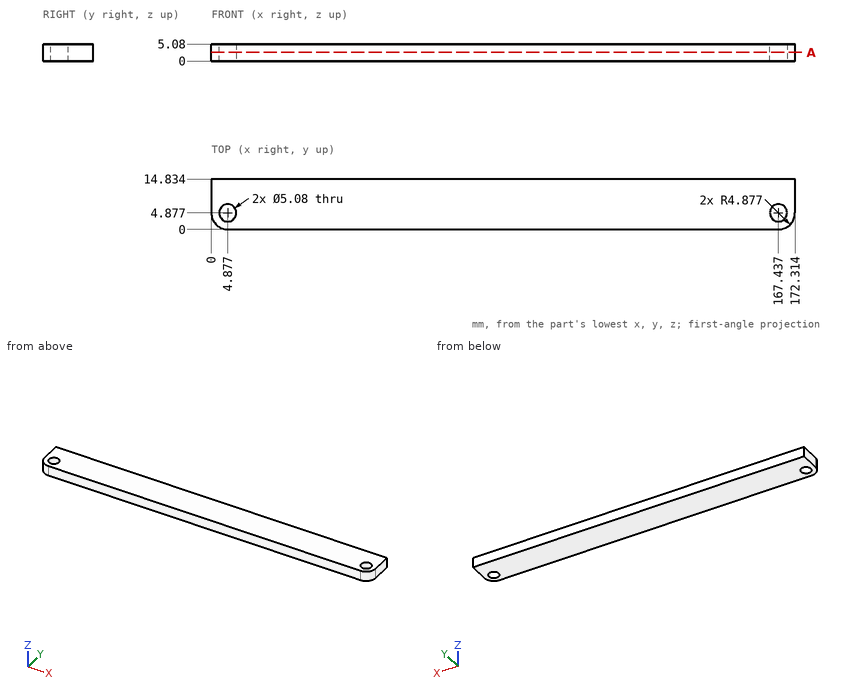
The drawing under review shows one solid part. Ordinate dimensions are in mm from its lowest x, y, z. Coordinates: 2 decimals unless noted, no trailing zeros. Order: outer loops, then holes, each group sorted by start corner. A loop starts at its lowest first (then second) coordinate and runs counter-clockwise, first axis right, second up. Notation, with made-up numbers: (47, 87.5) -> (89, 87.5) arc R18 ccw to (89, 99.5) -> close; hole circle Ø11 at (74.25, 46). An arc over 180 degrees is marked (long way). Use CSV: the item, a comma, the result in double quotes. Start each with the question number.
Item 1: Wall thickness on probe 1 along X at (y, z) = (3.5, 0.65) (1 decimal); probe 2 along X at (y, z) = (5.75, 1.85) (1 decimal); probe 3 along X at (y, z) = (1, 3.7) (1 decimal): over which ranges is each line inside the solid? List them lowest first.
Item 2: Insertion check: pin 1 (1 mm diameter, centred on y = 4, z = 4, fed in from -X) (1 decimal); pin 2 (3 mm diameter, centred on x = 99, y = 7.5, fed in from -Z); pin 3 (1 mm diameter, centred on y = 3, z = 4, fed in from -X). Each pin has a flat end and moves straight along its axis. Give the tip position at first contact, or say it passes through.
Item 3: We need section A-A, the plane z = 2.6. Give the boundary of the cut face in (x, y).
Derived:
1,probe 1,"x = 0.2 to 2.7, 7 to 165.3, 169.6 to 172.1"
1,probe 2,"x = 0 to 2.5, 7.3 to 165.1, 169.8 to 172.3"
1,probe 3,"x = 1.9 to 170.4"
2,pin 1,"stops at x = 0"
2,pin 2,"stops at z = 0"
2,pin 3,"stops at x = 0.2"
3,outline,"(0, 4.88) arc R4.88 ccw to (4.88, 0) -> (167.44, 0) arc R4.88 ccw to (172.31, 4.88) -> (172.31, 14.83) -> (0, 14.83) -> close; hole circle Ø5.08 at (4.88, 4.88); hole circle Ø5.08 at (167.44, 4.88)"
